Could you check a few things on this model? Use its own coordinates, in mm. A direction names the side the tool comes from. Coordinates: 2 decimals unless noted, no trailing zeros. Order: outer loops, then holes, each group sorted by start corner. A loop starts at its lowest first (then second) coordinate and runs counter-clockwise, first axis right, second up.
```python
from build123d import *

# Parameters (mm, degrees)
F0_R     = 11.1125
F0_R_2   = 10.61
F1_DEPTH = 6.35
F2_R     = 2.54


with BuildPart() as f1:
    # F0 (on Top) → F1 (new body)
    with BuildSketch(Plane.XY):
        with BuildLine():
            ThreePointArc((12.029634049, -6.9453126307), (13.4173134113, -3.5951583713), (13.890625, 0))
            ThreePointArc((13.890625, 0), (13.4173134613, 3.5951581844), (12.0296342424, 6.9453122957))
            ThreePointArc((12.0296342424, 6.9453122957), (6.9453126033, 12.0296340648), (2.8e-09, 13.890625))
            ThreePointArc((2.8e-09, 13.890625), (-6.9453125381, 12.0296341025), (-12.0296341698, 6.9453124214))
            ThreePointArc((-12.0296341698, 6.9453124214), (-13.890625, 1.22e-08), (-12.029634182, -6.9453124002))
            ThreePointArc((-12.029634182, -6.9453124002), (-6.9453125499, -12.0296340956), (0, -13.890625))
            ThreePointArc((0, -13.890625), (6.9453124346, -12.0296341622), (12.029634049, -6.9453126307))
        make_face()
        Circle(F0_R, mode=Mode.SUBTRACT)
        with BuildLine():
            ThreePointArc((12.0296342424, 6.9453122957), (13.4173134613, 3.5951581844), (13.890625, 0))
            ThreePointArc((13.890625, 0), (13.4173134113, -3.5951583713), (12.029634049, -6.9453126307))
            Line((12.029634049, -6.9453126307), (16.0395121659, 0))
            Line((16.0395121659, 0), (12.0296342424, 6.9453122957))
        make_face()
        with BuildLine():
            ThreePointArc((2.8e-09, 13.890625), (6.9453126033, 12.0296340648), (12.0296342424, 6.9453122957))
            Line((12.0296342424, 6.9453122957), (8.019756083, 13.890625))
            Line((8.019756083, 13.890625), (2.8e-09, 13.890625))
        make_face()
        with BuildLine():
            Line((8.019756083, -13.890625), (12.029634049, -6.9453126307))
            ThreePointArc((12.029634049, -6.9453126307), (6.9453124346, -12.0296341622), (0, -13.890625))
            Line((0, -13.890625), (8.019756083, -13.890625))
        make_face()
        Polygon((16.0395121659, 0), (12.029634049, -6.9453126307), (8.019756083, -13.890625), (16.0395121659, -27.78125), (32.0790243318, -27.78125), (40.0987804148, -13.890625), (32.0790243318, 0), align=None)
        with Locations((24.0592682489, -13.890625)):
            Circle(F0_R_2, mode=Mode.SUBTRACT)
        with BuildLine():
            ThreePointArc((-12.0296341698, 6.9453124214), (-6.9453125381, 12.0296341025), (2.8e-09, 13.890625))
            Line((2.8e-09, 13.890625), (-8.019756083, 13.890625))
            Line((-8.019756083, 13.890625), (-12.0296341698, 6.9453124214))
        make_face()
        with BuildLine():
            ThreePointArc((12.0296340896, 20.8359374397), (6.945312471, 15.7516158588), (2.8e-09, 13.890625))
            Line((2.8e-09, 13.890625), (8.019756083, 13.890625))
            Line((8.019756083, 13.890625), (12.0296340896, 20.8359374397))
        make_face()
        with BuildLine():
            Line((-8.019756083, 13.890625), (2.8e-09, 13.890625))
            ThreePointArc((2.8e-09, 13.890625), (-6.9453126113, 15.7516159398), (-12.0296342543, 20.8359377249))
            Line((-12.0296342543, 20.8359377249), (-8.019756083, 13.890625))
        make_face()
        with BuildLine():
            ThreePointArc((-12.0296342543, 20.8359377249), (-6.9453126113, 15.7516159398), (2.8e-09, 13.890625))
            ThreePointArc((2.8e-09, 13.890625), (6.945312471, 15.7516158588), (12.0296340896, 20.8359374397))
            ThreePointArc((12.0296340896, 20.8359374397), (13.4173134218, 24.186091668), (13.890625, 27.78125))
            ThreePointArc((13.890625, 27.78125), (13.4173134908, 31.3764080746), (12.0296343561, 34.7265620987))
            ThreePointArc((12.0296343561, 34.7265620987), (6.9453127227, 39.8108839959), (5.09e-08, 41.671875))
            ThreePointArc((5.09e-08, 41.671875), (-6.9453124478, 39.8108841546), (-12.0296340896, 34.7265625603))
            ThreePointArc((-12.0296340896, 34.7265625603), (-13.890625, 27.7812501647), (-12.0296342543, 20.8359377249))
        make_face()
        with Locations((0, 27.78125)):
            Circle(F0_R_2, mode=Mode.SUBTRACT)
        with BuildLine():
            Line((-8.019756083, -13.890625), (0, -13.890625))
            ThreePointArc((0, -13.890625), (-6.9453125499, -12.0296340956), (-12.029634182, -6.9453124002))
            Line((-12.029634182, -6.9453124002), (-8.019756083, -13.890625))
        make_face()
        with BuildLine():
            ThreePointArc((-12.029634182, -6.9453124002), (-13.890625, 1.22e-08), (-12.0296341698, 6.9453124214))
            Line((-12.0296341698, 6.9453124214), (-16.0395121659, 0))
            Line((-16.0395121659, 0), (-12.029634182, -6.9453124002))
        make_face()
        with BuildLine():
            Line((-16.0395121659, 27.78125), (-12.0296342543, 20.8359377249))
            ThreePointArc((-12.0296342543, 20.8359377249), (-13.890625, 27.7812501647), (-12.0296340896, 34.7265625603))
            Line((-12.0296340896, 34.7265625603), (-16.0395121659, 27.78125))
        make_face()
        with BuildLine():
            ThreePointArc((13.890625, 27.78125), (13.4173134218, 24.186091668), (12.0296340896, 20.8359374397))
            Line((12.0296340896, 20.8359374397), (16.0395121659, 27.78125))
            Line((16.0395121659, 27.78125), (12.0296343561, 34.7265620987))
            ThreePointArc((12.0296343561, 34.7265620987), (13.4173134908, 31.3764080746), (13.890625, 27.78125))
        make_face()
        Polygon((-8.019756083, -13.890625), (-12.029634182, -6.9453124002), (-16.0395121659, 0), (-32.0790243318, 0), (-40.0987804148, -13.890625), (-32.0790243318, -27.78125), (-16.0395121659, -27.78125), align=None)
        with Locations((-24.0592682489, -13.890625)):
            Circle(F0_R_2, mode=Mode.SUBTRACT)
        with BuildLine():
            Line((-8.019756083, 41.671875), (-12.0296340896, 34.7265625603))
            ThreePointArc((-12.0296340896, 34.7265625603), (-6.9453124478, 39.8108841546), (5.09e-08, 41.671875))
            Line((5.09e-08, 41.671875), (-8.019756083, 41.671875))
        make_face()
        with BuildLine():
            Line((8.019756083, 41.671875), (5.09e-08, 41.671875))
            ThreePointArc((5.09e-08, 41.671875), (6.9453127227, 39.8108839959), (12.0296343561, 34.7265620987))
            Line((12.0296343561, 34.7265620987), (8.019756083, 41.671875))
        make_face()
    extrude(amount=F1_DEPTH)

    # F2
    f2_edges = [f1.edges().sort_by_distance(p)[0] for p in [
        (-8.019756, -13.890625, 3.175),
        (8.019756, -13.890625, 3.175),
        (16.039512, -27.78125, 3.175),
        (32.079024, -27.78125, 3.175),
        (40.09878, -13.890625, 3.175),
        (-16.039512, -27.78125, 3.175),
        (-32.079024, -27.78125, 3.175),
        (-40.09878, -13.890625, 3.175),
        (32.079024, 0, 3.175),
        (16.039512, 0, 3.175),
        (16.039512, 27.78125, 3.175),
        (8.019756, 41.671875, 3.175),
        (-8.019756, 41.671875, 3.175),
        (8.019756, 13.890625, 3.175),
        (-16.039512, 27.78125, 3.175),
        (-8.019756, 13.890625, 3.175),
        (-16.039512, 0, 3.175),
        (-32.079024, 0, 3.175),
    ]]
    fillet(f2_edges, radius=F2_R)


solid = f1.part
```
Item 1: Suppose I cut it at D-D (y = 9). List the corners of the cut face in (x, z) for me, and give its area (3 significant figures).
Item 2: Which directions (+Z, -Z, +X, -X, +Y, -Y) give clear straight access to the entire face, cutting with the end or side of a thin tool? Please do faces 5 (the face through (12, 7, 3)), 6 (the face through (0, -13.891, 3)), 7 (the face through (10.6, 3.34, 3.13)), 8 (the face through (-12.08, 20.92, 3.13)), 9 (the face through (-36.043, -6.866, 3.131)).
Item 3: Suppose I cut it at A-A (x = 0). List the corners of the cut face in (y, z) for me.
Item 4: Suppose I cut it at C-C (x = 27.5). List the corners of the cut face in (y, z) for me, and give its area (3 significant figures).
Item 5: I need wall thicknesses on line 1 (Y direction, x = 0, z = 5); line 2 (Y direction, x = 3, z = 3.5); line 3 (X direction, y = -4.5, z = 5.75). Which ranges of each line are inside material? Lowest first, please.
Item 6: Suppose I cut it at B-B (y = -17). List the corners of the cut face in (x, z) for me, and give its area (3 significant figures).
Item 7: Thinking about a two-plate mould opening in Y: for faces 1 (the face through (-36.135, -20.756, 3.131)), 2 (the face through (16.22, 0.35, 3.22)), 3 (the face through (0, 41.672, 3)), 4 (the face through (-39.706, -13.872, 3.219)), which applies, +Y half, -Y half, draft (parallel to the pull), parting line (faces both ways), or undercut?
Item 8: For pin 1 Ø3 at (x, z) = (0, 4.5) entering from -Y; pin 2 Ø13.5 at (x, y) = (0, 0) entering from -Z; pin 3 Ø1.5 at (y, z) = (17, 2.5) entering from -X; pin 4 Ø3 at (x, z) = (25, 3) entering from +Y, each with a flat end and sliding along its axis, tell me the tip position at first contact or that it passes through.
Geometry results:
1. outline: (-10.84, 0) - (-6.52, 0) - (-6.52, 6.35) - (-10.84, 6.35) - close; (6.52, 0) - (10.84, 0) - (10.84, 6.35) - (6.52, 6.35) - close
1. area: 54.9 mm2
2. face 5: +Z, -Z, +X
2. face 6: +Z, -Z, -Y
2. face 7: +Z, -Z
2. face 8: +Z, -Z, -X
2. face 9: +Z, -Z, -X, +Y
3. outline: (-13.89, 0) - (-11.11, 0) - (-11.11, 6.35) - (-13.89, 6.35) - close; (11.11, 0) - (17.17, 0) - (17.17, 6.35) - (11.11, 6.35) - close; (38.39, 0) - (41.67, 0) - (41.67, 6.35) - (38.39, 6.35) - close
4. outline: (-27.78, 0) - (-23.93, 0) - (-23.93, 6.35) - (-27.78, 6.35) - close; (-3.85, 0) - (0, 0) - (0, 6.35) - (-3.85, 6.35) - close
4. area: 48.9 mm2
5. line 1: y = -13.89 to -11.11, 11.11 to 17.17, 38.39 to 41.67
5. line 2: y = -13.89 to -10.7, 10.7 to 17.6, 37.96 to 41.67
5. line 3: x = -34.68 to -29, -19.12 to -10.16, 10.16 to 19.12, 29 to 34.68
6. outline: (-38.3, 0) - (-34.2, 0) - (-34.2, 6.35) - (-38.3, 6.35) - close; (-13.92, 0) - (-9.81, 0) - (-9.81, 6.35) - (-13.92, 6.35) - close; (9.81, 0) - (13.92, 0) - (13.92, 6.35) - (9.81, 6.35) - close; (34.2, 0) - (38.3, 0) - (38.3, 6.35) - (34.2, 6.35) - close
6. area: 104 mm2
7. face 1: -Y half
7. face 2: undercut
7. face 3: +Y half
7. face 4: parting line
8. pin 1: stops at y = -13.89
8. pin 2: passes through
8. pin 3: stops at x = -10.25
8. pin 4: stops at y = 0
